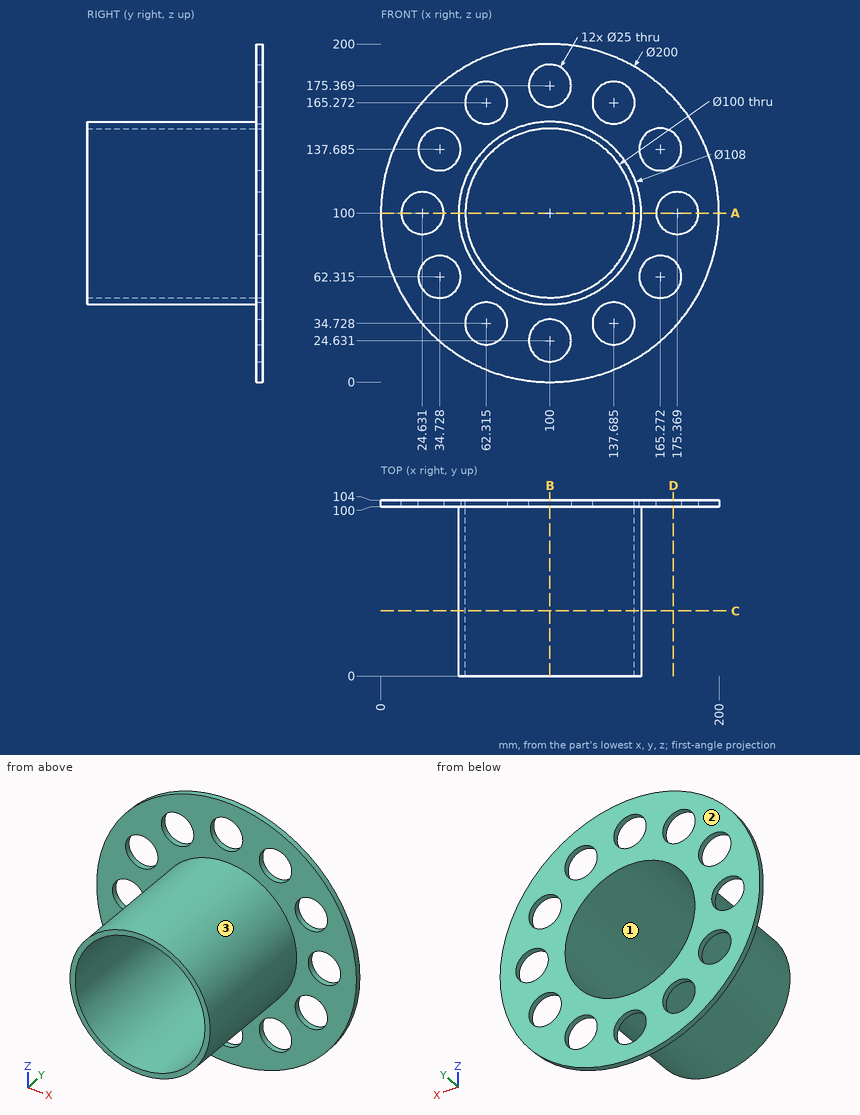
Could you check a few things on this drawing? It's one solid part, dimensions in mm from its lowest x, y, z. Give positions to 0.01 mm unless a question says otherwise; leave off trailing zeros. Order: outer loops, then holes, each group sorted by start corner. A loop starts at its lowest first (then second) coordinate and runs counter-clockwise, first axis right, second up. Notation, with made-up numbers: (2, 8.5) - (27, 8.5) arc R15 cw to (27, 25.5) - close; hole circle Ø2 at (-33.5, 15.5). An arc over 180 degrees is marked (long way). Answer as a JSON object with one key per item and string values. Group by question number.
Item 1: Please list where these lines run through material, in increasing order: probe 1 along Z at (x, y) = (100, 101.35); probe 2 along Z at (x, y) = (100, 54); probe 3 along Z at (x, y) = (66, 89.5).
Item 2: For P1, Ø3, axis at x = 118, y = 66.5, coming from the -Z side; P2, Ø1.5, axis at x = 74, y = 15, coming from the +Z side; P3, Ø2, axis at y = 31.5, z = 116, coming from the +X side (1 decimal), each with a flat end and sliding along its axis, tell me the tip position at first contact or that it passes through.
Item 3: If we section it at D-D on x = 173: Please give me the cut outline in (y, z) (1 decimal).
Item 4: If we mould it in two halves opening along Z, with no side actions, what happens to the marked faces 1, 2 and 3? For each: pulls with the +Z half, pulls with the -Z half, needs draft (parallel to the pull), parting line crosses it, or undercut.
Item 5: If we section it at C-C on y = 38.5: Please give me the cut outline in (x, z), and give its area (3 significant figures).
Item 6: If we section it at A-A on z = 100: Please give me the cut outline in (x, y).
Item 7: If we section it at B-B on x = 100: Please give me the cut outline in (y, z), and give its area (3 significant figures).
Result set:
{
 "1": {"probe 1": "0 to 12.13, 37.13 to 50, 150 to 162.87, 187.87 to 200", "probe 2": "46 to 50, 150 to 154", "probe 3": "58.05 to 63.34, 136.66 to 141.95"},
 "2": {"P1": "z = 48.58", "P2": "z = 147.73", "P3": "x = 151.9"},
 "3": {"outline": "(100, 31.7) - (104, 31.7) - (104, 52.5) - (100, 52.5) - close; (100, 72.1) - (104, 72.1) - (104, 87.7) - (100, 87.7) - close; (100, 112.3) - (104, 112.3) - (104, 127.9) - (100, 127.9) - close; (100, 147.5) - (104, 147.5) - (104, 168.3) - (100, 168.3) - close"},
 "4": {"face 1": "undercut", "face 2": "needs draft", "face 3": "parting line crosses it"},
 "5": {"outline": "circle Ø108 at (100, 100); hole circle Ø100 at (100, 100)", "area": "1,310 mm²"},
 "6": {"outline": "(0, 100) - (12.13, 100) - (12.13, 104) - (0, 104) - close; (37.13, 100) - (46, 100) - (46, 0) - (50, 0) - (50, 104) - (37.13, 104) - close; (150, 0) - (154, 0) - (154, 100) - (162.87, 100) - (162.87, 104) - (150, 104) - close; (187.87, 100) - (200, 100) - (200, 104) - (187.87, 104) - close"},
 "7": {"outline": "(0, 46) - (100, 46) - (100, 37.13) - (104, 37.13) - (104, 50) - (0, 50) - close; (0, 150) - (104, 150) - (104, 162.87) - (100, 162.87) - (100, 154) - (0, 154) - close; (100, 0) - (104, 0) - (104, 12.13) - (100, 12.13) - close; (100, 187.87) - (104, 187.87) - (104, 200) - (100, 200) - close", "area": "1,000 mm²"}
}
